from build123d import *

# Parameters (mm, degrees)
SKETCH1_R                       = 127
BOSS_EXTRUDE1_DEPTH             = 7.9375
F_5_32_0_15625_DIAMETER_HOLE2_D = 3.96875


with BuildPart() as part:
    # Sketch1 → Boss-Extrude1 (new body)
    with BuildSketch(Plane(origin=(0, 0, 0), x_dir=(1, 0, 0), z_dir=(0, 1, 0))):
        with Locations(Location((0, 0, 0), (0, 0, 270))):
            Circle(SKETCH1_R)
    extrude(amount=BOSS_EXTRUDE1_DEPTH)

    # 5/32 (0.15625) Diameter Hole2 (through all)
    with Locations(Plane(origin=(0, 7.9375, 0), x_dir=(1, 0, 0), z_dir=(0, 1, 0))):
        with Locations((31.75, 31.75), (-31.75, -31.75), (-31.75, 31.75), (31.75, -31.75), (0, 0)):
            Hole(F_5_32_0_15625_DIAMETER_HOLE2_D / 2)


solid = part.part
Geometry check sheet. Reference: the model listing, model coordinates, mm. Give positions to 0.01 mm unless a question says otherwise; leave off trailing zeros. Loops run counter-clockwise (first coordinate to the right, second up) from the corner with the lowest first, then second, coordinate; pieces in that order, holes last. Notation, with made-up numbers: M 83,33.25 L 106,33.25 A13 cw 106,48.25 Z; hole C -30,-33.75 d8. An arc over 180 degrees is marked long. Answer as a JSON object with one key per item and string values. Group by question number.
Item 1: Material ranges on L1, parallel to Z at x = -31.5, y = 7; L2, parallel to X at y = 4.25, z = -31.75; L3, parallel to X at y = 5, z = -90.5, recorded low to high.
Item 2: Sectioned sample at A-A on y = 5.5. Record the boundary of the cut face in (x, z).
Item 3: Sectioned sample at B-B on x = 48. Record the boundary of the cut face in (y, z).
Item 4: Sectioned sample at C-C on z = 72.5. Record the boundary of the cut face in (x, y).
Item 5: Gauge pin test, flat ends, axial feed: pin 1 (2 mm diameter, centred on x = 36.5, y = 4.5, fed in from +Z); pin 2 (2 mm diameter, centred on x = 19.5, y = 1, fed in from -Z); pin 3 (1 mm diameter, centred on x = 101.5, y = 6, fed in from +Z). Record the tip position at first contact, or that the pin passes through.
Findings below:
{
 "1": {"L1": "-123.03 to -33.72, -29.78 to 29.78, 33.72 to 123.03", "L2": "-122.97 to -33.73, -29.77 to 29.77, 33.73 to 122.97", "L3": "-89.1 to 89.1"},
 "2": {"outline": "C 0,0 d254; hole C -31.75,-31.75 d3.97; hole C -31.75,31.75 d3.97; hole C 0,0 d3.97; hole C 31.75,-31.75 d3.97; hole C 31.75,31.75 d3.97"},
 "3": {"outline": "M 0,-117.58 L 7.94,-117.58 L 7.94,117.58 L 0,117.58 Z"},
 "4": {"outline": "M -104.27,0 L 104.27,0 L 104.27,7.94 L -104.27,7.94 Z"},
 "5": {"pin 1": "z = 121.94", "pin 2": "z = -125.65", "pin 3": "z = 76.99"}
}
